For this review, take the finished solid that the model builds, in its own axes (mm). A direction names the side the tool comes from. Give positions to 0.01 mm unless a question says otherwise; leave off trailing zeros. Write each loop counter-clockwise with the first axis right and the second up, starting at its lowest first coordinate (ties: lowest second). Pieces come first, ordered by that corner, then holes. Notation, with made-up numbers: M -23.5,84.25 L -7.5,84.25 A32 ccw -7.5,111.25 Z; hole C 26.25,42.25 d11. An arc over 180 degrees is marked long. Answer as a JSON object with one key per item and string values. Group by question number.
Autodesk Inventor part; units mm, degrees
ref_plane "Work Plane3" through (167.8, -16.921, -48) normal (-1, 0, 0) x (0, 0, 1)
ref_plane "YZ Plane" through (0, 0, 0) normal (1, 0, 0) x (0, 1, 0)
ref_plane "XZ Plane" through (0, 0, 0) normal (0, 1, 0) x (-1, 0, 0)
ref_plane "Work Plane1" through (182.8, -16.921, -7.958) normal (0, -1, 0) x (0, 0, -1)
ref_plane "Work Plane2" through (182.8, -6.9868, -42.1222) normal (1, 0, 0) x (0, 0, -1)
sketch "Sketch1" plane through (182.8, -6.9868, -42.1222) normal (1, 0, 0) x (0, 0, -1)
  arc A0 (5.0194, 6.9868) -> (5.8778, 5.8182) centre (7.8778, 8.1868) ccw
  line L0 (-9.7772, 6.9868) -> (5.0194, 6.9868)
  arc A1 (-7.9865, 5.8774) -> (-9.7772, 6.9868) centre (-9.7772, 4.9868) ccw
  line L1 (-7.9865, 5.8774) -> (-0.1222, -9.9342)
  line L2 (-0.1222, -9.9342) -> (5.8778, -9.9342)
  line L3 (5.8778, -9.9342) -> (5.8778, 5.8182)
  line L4 (-42.1222, 6.9868) -> (-42.1222, -9.9342)
  line L5 (-42.1222, -9.9342) -> (-34.1642, -9.9342)
  line L6 (-34.1642, -9.9342) -> (-26.2998, 5.8774)
  arc A2 (-24.5091, 6.9868) -> (-26.2998, 5.8774) centre (-24.5091, 4.9868) ccw
  line L7 (-42.1222, 6.9868) -> (-24.5091, 6.9868)
  circle A3 centre (-17.1432, -9.9342) radius 15.24 construction
  line L8 (-17.1432, -9.9342) -> (-17.1432, -20.9232) construction
  line L9 (-17.1432, -9.9342) -> (-6.1542, -9.9342) construction
  line L10 (-0.1222, -9.9342) -> (-8.2255, -25.1742)
  line L11 (-0.1222, -9.9342) -> (17.1381, -9.9342) construction
  line L12 (-8.2255, -25.1742) -> (-17.1432, -25.1742)
  line L13 (-17.1432, -25.1742) -> (-17.1432, -28.1742)
  line L14 (-17.1432, -28.1742) -> (5.8778, -28.1742)
  line L15 (5.8778, -28.1742) -> (5.8778, -9.9342)
  line L16 (-0.1222, -9.9342) -> (5.8778, -9.9342)
  dimension "d0" = 90
  dimension "d1" = 118
  dimension "d2" = 3
  dimension "d3" = 90
ref_plane "Work Plane3" through (167.8, -16.921, -48) normal (-1, 0, 0) x (0, 0, 1)
extrude "Extrusion1" add sketch "Sketch1" against normal up to surface (15 mm away) contours L15 L14 L13 L12 L10 L2
sketch "Sketch2" plane through (182.8, -35.161, -48) normal (0, -1, 0) x (1, 0, 0)
  circle A0 centre (-7.5, 3) radius 1.45
  point P0 (-182.8, 48)
hole "Hole1" at (175.3, -35.161, -45) direction (0, 1, 0) diameter 3.5 end through all counterbore diameter 6 counterbore depth 6.5
mirror "Mirror1" about plane through (182.8, -35.161, -24.979) normal (0, 0, 1) of "Extrusion1", "Hole1"
ref_plane "Work Plane4" through (119.0599, -16.9209, 25.2669) normal (0.9026, 0, -0.4305) x (0.4305, 0, 0.9026)
sketch "Sketch3" plane through (119.0599, -16.9209, 25.2669) normal (0.9026, 0, -0.4305) x (0.4305, 0, 0.9026)
  circle A0 centre (0, 0) radius 12.5
  circle A1 centre (0, 0) radius 5.5
  point P0 (-74.0621, -16.9209)
  dimension "d13" = 11
extrude "Extrusion2" cut sketch "Sketch3" along normal through all contours A1
properties part number "30_CUBE_openSIM_Lensfixation"
Item 1: Consider section A-A (z = -45). Give the boundary of the cut face in (x, y).
Item 2: Machinability: for faces 1 (the cylindrical face through (177.8, -31.9, -3.3)), 2 (the flat face through (175, -35.161, -25)), 3 (the flat face through (175.405, -24.648, -12.066)), which of the approach directions +Z, -Z, +X, -X, +Y, -Y give a long, thin tool a straight path to every point of the face, cutting with its end or side? Answer none if there is none.
Item 3: Consider section C-C (x = 174.5). State how many separate pieces and enclosed holes the cut face has, plus the area to 3 significant figures.
Item 4: To check wall thickness, follow probe 1 along Z at (x, y) = (175.3, -24); probe 2 along Z at (x, y) = (175.3, -24.5); probe 3 along X at (y, z) = (-32.5, -45). State the ranges of each line that lie inside material, in increasing order.
Item 5: Consider section B-B (y = -25.75). Give the boundary of the cut face in (x, z), plus the area to 3 significant figures.
Item 6: Draft analysis for pull direction Z (two halves, no side actions). For faces 4 (the flat face through (177, -28.661, -6)), 5 (the flat face through (177, -16.921, -44)), 6 (the flat face through (175, -26, -48)), 7 (the flat face through (175.405, -24.434, -38.005)), state which applies: released by +Z, released by -Z, zero draft, split by the parting line, or undercut.
Item 7: Consider section D-D (z = -23). Give the boundary of the cut face in (x, y), plus the area to 3 significant figures.
Item 8: Insertion check: P1, Ø4, axis at x = 175.3, z = -4.958, coming from the -Y side; P2, Ø3, axis at x = 175.3, z = -45, coming from the +Y side. Each pin has a flat end and moves straight along its axis. Give the tip position at first contact, or say it passes through.
Result set:
{
 "1": {"outline": "M 167.8,-35.16 L 172.3,-35.16 L 172.3,-28.66 L 173.55,-28.66 L 173.55,-16.92 L 167.8,-16.92 Z; M 177.05,-28.66 L 178.3,-28.66 L 178.3,-35.16 L 182.8,-35.16 L 182.8,-16.92 L 177.05,-16.92 Z"},
 "2": {"face 1": "-Y", "face 2": "+Z, -Z, +X, -X, -Y", "face 3": "+X, -X, +Y"},
 "3": {"separate pieces": "3", "enclosed holes": "0", "area": "287 mm^2"},
 "4": {"probe 1": "z = -48 to -46.75, -43.25 to -38.24, -11.72 to -6.71, -3.21 to -1.96", "probe 2": "z = -48 to -46.75, -43.25 to -37.97, -11.99 to -6.71, -3.21 to -1.96", "probe 3": "x = 167.8 to 172.3, 178.3 to 182.8"},
 "5": {"outline": "M 167.8,-48 L 182.8,-48 L 182.8,-37.31 L 167.8,-37.31 Z; M 167.8,-12.65 L 182.8,-12.65 L 182.8,-1.96 L 167.8,-1.96 Z; hole C 175.3,-45 d3.5; hole C 175.3,-4.96 d3.5", "area": "302 mm^2"},
 "6": {"face 4": "undercut", "face 5": "zero draft", "face 6": "released by -Z", "face 7": "undercut"},
 "7": {"outline": "M 167.8,-35.16 L 182.8,-35.16 L 182.8,-32.16 L 167.8,-32.16 Z", "area": "45.0 mm^2"},
 "8": {"P1": "stops at y = -28.66", "P2": "passes through"}
}
